Can you work these out from the model? Positions are in its coordinate system, mm. A direction names the side the tool comes from. Round coordinates to 2 decimals unless told otherwise and drop trailing zeros. Write each loop counter-clockwise with the first axis right and the second up, starting at its lowest first coordinate (ties: lowest second). Pieces come first, ordered by that corner, then holes.
Q1. I'm going to push flat-ended pins straight in: pin 1 Ø1.9 at (x, z) = (27, 1) entering from -Y; pin 2 Ø2 at (x, z) = (-6, 4.5) entering from +Y (1 decimal); pin 3 Ø1.5 at (x, y) = (4, 36) entering from +Z. Where does each tip first touch, or does it pass through?
Q2. If we section it at C-C (y = 21.57): Please give me the cut outline in (x, z).
Q3. If we section it at A-A (x = 3.5): Please give me the cut outline in (y, z).
Q4. Please list where these lines run through material, in increasing order: line 1 along Z through (x, y) = (26, 75.5); line 2 along Y through (x, z) = (3, 1); line 3 along X through (y, z) = (5.5, 5.5).
Q5. For faces 4 (the flat face through (-28, 24.87, 1)), 5 (the flat face through (5, -1, 1.7)), 6 (the flat face through (28, 59.13, 1)), which set-ups out of +Z, -Z, +X, -X, +Y, -Y let a thin tool reach every point of the face, with its end or its side?
Q6. If we section it at B-B (y = 40.5): Please give me the cut outline in (x, z).
Q7. We'd pull the mould along Y, two halves only. Please class faces 1 (the flat face through (28, 24.87, 1)), 2 (the flat face through (13, 3, 5)), 3 (the flat face through (0, 84, 1)): +Y half, -Y half, draft (parallel to the pull), parting line (faces both ways), or undercut.
from build123d import *

# Parameters (mm, degrees)
PAD_DEPTH       = 1.7
SKETCH006_W     = 15.05
SKETCH006_H     = 11.12
PAD005_DEPTH    = 6.31
SKETCH012_W     = 11.05
SKETCH012_H     = 0.1
POCKET001_DEPTH = 3.7
FILLET002_R     = 0.2
FILLET003_R     = 0.2
FILLET010_R     = 0.5


with BuildPart() as part:
    # Sketch → Pad (new body)
    with BuildSketch(Plane.XY):
        with BuildLine():
            Line((0, 0), (30, 0))
            Line((30, 0), (30, 1))
            Line((30, 1), (31, 1))
            Line((31, 1), (31, 18.27))
            Line((31, 18.27), (24.4, 18.27))
            ThreePointArc((24.4, 24.87), (21.1, 21.57), (24.4, 18.27))
            Line((24.4, 24.87), (31, 24.87))
            Line((31, 24.87), (31, 59.13))
            Line((31, 59.13), (24.4, 59.13))
            ThreePointArc((24.4, 65.73), (21.1, 62.43), (24.4, 59.13))
            Line((24.4, 65.73), (31, 65.73))
            Line((31, 65.73), (31, 83))
            Line((30, 83), (31, 83))
            Line((30, 84), (30, 83))
            Line((30, 84), (0, 84))
            Line((0, 84), (-30, 84))
            Line((-30, 84), (-30, 83))
            Line((-30, 83), (-31, 83))
            Line((-31, 83), (-31, 65.73))
            Line((-31, 65.73), (-24.4, 65.73))
            ThreePointArc((-24.4, 59.13), (-21.1, 62.43), (-24.4, 65.73))
            Line((-24.4, 59.13), (-31, 59.13))
            Line((-31, 59.13), (-31, 24.87))
            Line((-31, 24.87), (-24.4, 24.87))
            ThreePointArc((-24.4, 18.27), (-21.1, 21.57), (-24.4, 24.87))
            Line((-24.4, 18.27), (-31, 18.27))
            Line((-31, 18.27), (-31, 1))
            Line((-31, 1), (-30, 1))
            Line((-30, 1), (-30, 0))
            Line((-30, 0), (0, 0))
        make_face()
    extrude(amount=PAD_DEPTH)

    # Sketch006 → Pad005 (new body)
    with BuildSketch(Plane.XY.offset(1.7)):
        with Locations((5.475, 2.86)):
            Rectangle(SKETCH006_W, SKETCH006_H)
    extrude(amount=PAD005_DEPTH)

    # Sketch012 → Pocket001 (cut)
    with BuildSketch(Plane.XZ.offset(2.7)):
        with BuildLine():
            Line((-2.05, 1.7), (-2.05, 3.2))
            ThreePointArc((-0.55, 1.7), (-0.98934, 2.76066), (-2.05, 3.2))
            Line((-2.05, 1.7), (-0.55, 1.7))
        make_face()
        with BuildLine():
            Line((13, 3.2), (13, 1.7))
            Line((13, 1.7), (11.5, 1.7))
            ThreePointArc((13, 3.2), (11.93934, 2.76066), (11.5, 1.7))
        make_face()
        with BuildLine():
            Line((-1.55, 7.51), (12.5, 7.51))
            Line((12.5, 7.51), (12.5, 3.7))
            ThreePointArc((12.5, 3.7), (11.43934, 3.26066), (11, 2.2))
            Line((11, 2.2), (-0.05, 2.2))
            ThreePointArc((-0.05, 2.2), (-0.48934, 3.26066), (-1.55, 3.7))
            Line((-1.55, 3.7), (-1.55, 7.51))
        make_face()
        with Locations((5.44813, 5.25)):
            Rectangle(SKETCH012_W, SKETCH012_H, mode=Mode.SUBTRACT)
    extrude(amount=-POCKET001_DEPTH, mode=Mode.SUBTRACT)

    # Fillet002
    fillet002_edges = [part.edges().sort_by_distance(p)[0] for p in [
        (13, 2.86, 8.01),
    ]]
    fillet(fillet002_edges, radius=FILLET002_R)

    # Fillet003
    fillet003_edges = [part.edges().sort_by_distance(p)[0] for p in [
        (-2.05, 2.86, 8.01),
    ]]
    fillet(fillet003_edges, radius=FILLET003_R)

    # Fillet010
    fillet010_edges = [part.edges().sort_by_distance(p)[0] for p in [
        (-0.55, -1.35, 1.7),
        (-2.05, -0.85, 3.2),
        (13, -0.85, 3.2),
        (11.5, -1.35, 1.7),
    ]]
    fillet(fillet010_edges, radius=FILLET010_R)


solid = part.part
A:
1. pin 1: stops at y = 0
1. pin 2: passes through
1. pin 3: stops at z = 1.7
2. outline: (-21.1, 0) - (21.1, 0) - (21.1, 1.7) - (-21.1, 1.7) - close
3. outline: (-2.7, 1.7) - (0, 1.7) - (0, 0) - (84, 0) - (84, 1.7) - (8.42, 1.7) - (8.42, 8.01) - (-2.7, 8.01) - (-2.7, 7.51) - (1, 7.51) - (1, 5.3) - (-2.7, 5.3) - (-2.7, 5.2) - (1, 5.2) - (1, 2.2) - (-2.7, 2.2) - close
4. line 1: z = 0 to 1.7
4. line 2: y = 0 to 84
4. line 3: x = -2.05 to 13
5. face 4: +Z, -Z, -X
5. face 5: -Z, +X, -X, -Y
5. face 6: +Z, -Z, +X
6. outline: (-31, 0) - (31, 0) - (31, 1.7) - (-31, 1.7) - close
7. face 1: undercut
7. face 2: draft
7. face 3: +Y half
